```python
from build123d import *

# Parameters (mm, degrees)
SKETCH1_R           = 10.85
SKETCH1_R_2         = 4.5
SKETCH1_R_3         = 1.55
BOSS_EXTRUDE1_DEPTH = 7
SKETCH2_R           = 1.55
BOSS_EXTRUDE2_DEPTH = 3


with BuildPart() as part:
    # Sketch1 → Boss-Extrude1 (new body)
    with BuildSketch(Plane.XY):
        Circle(SKETCH1_R)
        Circle(SKETCH1_R_2, mode=Mode.SUBTRACT)
        with Locations((-7.8, 0)):
            Circle(SKETCH1_R_3, mode=Mode.SUBTRACT)
        with Locations((0, 7.8)):
            Circle(SKETCH1_R_3, mode=Mode.SUBTRACT)
        with Locations((7.8, 0)):
            Circle(SKETCH1_R_3, mode=Mode.SUBTRACT)
        with Locations((0, -7.8)):
            Circle(SKETCH1_R_3, mode=Mode.SUBTRACT)
    extrude(amount=BOSS_EXTRUDE1_DEPTH)

    # Sketch2 → Boss-Extrude2 (add)
    with BuildSketch(Plane.XY.offset(7)):
        with Locations((0, 7.8)):
            Circle(SKETCH2_R)
        with Locations((-7.8, 0)):
            Circle(SKETCH2_R)
        with Locations((0, -7.8)):
            Circle(SKETCH2_R)
        with Locations((7.799999915, 0.00162894)):
            Circle(SKETCH2_R)
    extrude(amount=-BOSS_EXTRUDE2_DEPTH)


solid = part.part
```
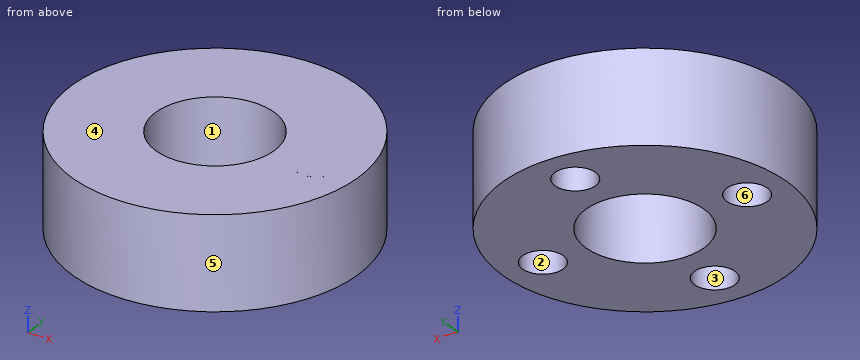
Part model, mm, in its own coordinate system. Face numbers are marked on the shaded views. A direction names the side the tool comes from. Round coordinates to 2 decimals unless told otherwise and drop trailing zeros. Write each loop counter-clockwise with the first axis right and the second up, starting at its lowest first coordinate (ties: lowest second). Pieces come first, ordered by that corner, then holes. Notation, with made-up numbers: (6.5, -2.5) -> (56.5, -2.5) arc R17 ccw to (56.5, 29.5) -> close; hole circle Ø11 at (71, -16). An arc over 180 degrees is marked (long way). Return JSON: item names as keys, results as strings. Group by question number.
Q1. Saw through at C-C on y = -1. Write the cut outline in (x, z), plus the area to 3 significant figures.
Q2. Which spindle directions (+Z, -Z, +X, -X, +Y, -Y) get a long thin tool onto all of the face, cutting with end or side? Do the marked faces 1, 2 and 3. Say none if no direction does.
Q3. Saw through at B-B on z = 1.25. Write the cut outline in (x, y), plus the area to 3 significant figures.
Q4. Mould opens along X. For the marked faces 4, 5 and 6 say: pulls with the +X half, pulls with the -X half, needs draft (parallel to the pull), parting line crosses it, or undercut.
Q5. Saw through at D-D on y = -7.8. Write the cut outline in (x, z).
Q6. Pin check, flat tips, straight feed: pin 1 (3 mm diameter, centred on x = -7.8, y = 0, fed in from -Z); pin 2 (2 mm diameter, centred on x = 5.5, z = 6, fed in from +Y); pin 3 (1.5 mm diameter, centred on x = -5.5, z = 3, fed in from -Y) (3 decimals); pin 4 (7 mm diameter, centred on x = 0, y = 0, fed in from -Z). Stop position of each tip, or through.
Q7. Probe L1, parallel to Y at x = 0, z = 3; L2, parallel to Y at x = -3, z = 3; L3, parallel to Y at x = 5.5, z = 5.5. List the from-to ranges inside material, lowest first. Write a range as [from, to].
Q8. Saw through at A-A on x = 7.8. Write the cut outline in (y, z).
Answer:
{
 "1": {"outline": "(-10.8, 0) -> (-8.98, 0) -> (-8.98, 4) -> (-6.62, 4) -> (-6.62, 0) -> (-4.39, 0) -> (-4.39, 7) -> (-10.8, 7) -> close; (4.39, 0) -> (6.62, 0) -> (6.62, 7) -> (4.39, 7) -> close; (6.62, 4) -> (8.98, 4) -> (8.98, 7) -> (6.62, 7) -> close; (8.98, 0) -> (10.8, 0) -> (10.8, 7) -> (8.98, 7) -> close", "area": "70.9 mm2"},
 "2": {"face 1": "+Z, -Z", "face 2": "none", "face 3": "-Z"},
 "3": {"outline": "circle Ø21.7 at (0, 0); hole circle Ø3.1 at (-7.8, 0); hole circle Ø9 at (0, 0); hole circle Ø3.1 at (0, -7.8); hole circle Ø3.1 at (0, 7.8); hole circle Ø3.1 at (7.8, 0)", "area": "276 mm2"},
 "4": {"face 4": "needs draft", "face 5": "parting line crosses it", "face 6": "undercut"},
 "5": {"outline": "(-7.54, 0) -> (-1.55, 0) -> (-1.55, 4) -> (1.55, 4) -> (1.55, 0) -> (7.54, 0) -> (7.54, 7) -> (-7.54, 7) -> close"},
 "6": {"pin 1": "z = 4", "pin 2": "y = 9.87", "pin 3": "y = -9.755", "pin 4": "through"},
 "7": {"L1": "[-10.85, -9.35], [-6.25, -4.5], [4.5, 6.25], [9.35, 10.85]", "L2": "[-10.43, -3.35], [3.35, 10.43]", "L3": "[-9.35, 9.35]"},
 "8": {"outline": "(-7.54, 0) -> (-1.55, 0) -> (-1.55, 7) -> (-7.54, 7) -> close; (-1.55, 4) -> (1.55, 4) -> (1.55, 0) -> (7.54, 0) -> (7.54, 7) -> (-1.55, 7) -> close"}
}
